Check sheet for the modelled part. Datum: model origin and axes. Units: mm. A direction names the side the tool comes from. Round coordinates to 2 decimals unless told otherwise and drop trailing zeros. Loops run counter-clockwise (first coordinate to the right, second up) from the corner with the lowest first, then second, coordinate; pieces in that order, holes last. Notation, with made-up numbers: (5, 47) - (31, 47) arc R26 ccw to (31, 64) - close; hole circle Ø4 at (85, 28.5). An arc over 180 degrees is marked (long way). Put each result on its own line as item: value.
```python
from build123d import *

# Parameters (mm, degrees)
SKETCH043_R     = 19
PAD026_DEPTH    = 3
PAD027_DEPTH    = 18.5
SKETCH045_W     = 5.4
SKETCH045_H     = 2
PAD028_DEPTH    = 1
SKETCH046_W     = 5.4
SKETCH046_H     = 2
PAD029_DEPTH    = 1
SKETCH047_W     = 5.4
SKETCH047_H     = 2
PAD030_DEPTH    = 1
SKETCH048_W     = 5.4
SKETCH048_H     = 2
PAD031_DEPTH    = 1
POCKET017_DEPTH = 5
CHAMFER_SIZE    = 1
CHAMFER001_SIZE = 1
CHAMFER002_SIZE = 1
CHAMFER003_SIZE = 1


with BuildPart() as part:
    # Sketch043 (on Face61 of Binder008) → Pad026 (new body)
    with BuildSketch(Plane.XY.offset(16.2)):
        with Locations((-83.63961, 83.63961)):
            Circle(SKETCH043_R)
    extrude(amount=PAD026_DEPTH)

    # Sketch044 (on Face2 of Pad026) → Pad027 (join)
    with BuildSketch(Plane(origin=(0, 0, 16.2), x_dir=(1, 0, 0), z_dir=(0, 0, -1))):
        Polygon((-92.9027091403, -78.1948880917), (-91.2056528655, -79.8919443665), (-87.3872762471, -76.0735677481), (-89.0843325219, -74.3765114732), align=None)
        Polygon((-79.8919443665, -76.0735677481), (-76.0735677481, -79.8919443665), (-74.3764965771, -78.1949029878), (-78.1948880917, -74.3765114732), align=None)
        Polygon((-92.9027199513, -89.0843217109), (-91.2056528655, -87.3872762471), (-87.3872762471, -91.2056528655), (-89.0843325219, -92.9027091403), align=None)
        Polygon((-79.8919443665, -91.2056528655), (-76.0735677481, -87.3872762471), (-74.3765262449, -89.0843472936), (-78.1948880917, -92.9027091403), align=None)
    extrude(amount=PAD027_DEPTH)

    # Sketch045 (on Face6 of Pad027) → Pad028 (join)
    with BuildSketch(Plane(origin=(-5.6568542495, -5.6568542495, 0), x_dir=(-0.7071067812, 0.7071067812, 0), z_dir=(0.7071067812, 0.7071067812, 0))):
        with Locations((118.2842712475, -1.3)):
            Rectangle(SKETCH045_W, SKETCH045_H)
    extrude(amount=PAD028_DEPTH)

    # Sketch046 (on Face11 of Pad028) → Pad029 (join)
    with BuildSketch(Plane(origin=(-89.2964645563, 89.2964645563, 0), x_dir=(0.7071067812, 0.7071067812, 0), z_dir=(0.7071067812, -0.7071067812, 0))):
        with Locations((0, -1.3)):
            Rectangle(SKETCH046_W, SKETCH046_H)
    extrude(amount=PAD029_DEPTH)

    # Sketch047 (on Face11 of Pad029) → Pad030 (join)
    with BuildSketch(Plane(origin=(-77.9827560573, 77.9827560573, 0), x_dir=(-0.7071067812, -0.7071067812, 0), z_dir=(-0.7071067812, 0.7071067812, 0))):
        with Locations((0, -1.3)):
            Rectangle(SKETCH047_W, SKETCH047_H)
    extrude(amount=PAD030_DEPTH)

    # Sketch048 (on Face15 of Pad030) → Pad031 (join)
    with BuildSketch(Plane(origin=(5.6568542495, 5.6568542495, 0), x_dir=(0.7071067812, -0.7071067812, 0), z_dir=(-0.7071067812, -0.7071067812, 0))):
        with Locations((-118.2842712475, -1.3)):
            Rectangle(SKETCH048_W, SKETCH048_H)
    extrude(amount=PAD031_DEPTH)

    # Sketch049 (on Face3 of Pad031) → Pocket017 (cut)
    with BuildSketch(Plane.XY.offset(19.2)):
        Polygon((-86.0396103068, 96.0396103068), (-81.2396103068, 96.0396103068), (-81.2396103068, 86.0396103068), (-71.2396103068, 86.0396103068), (-71.2396103068, 81.2396103068), (-81.2396103068, 81.2396103068), (-81.2396103068, 71.2396103068), (-86.0396103068, 71.2396103068), (-86.0396103068, 81.2396103068), (-96.0396103068, 81.2396103068), (-96.0396103068, 86.0396103068), (-86.0396103068, 86.0396103068), align=None)
    extrude(amount=-POCKET017_DEPTH, mode=Mode.SUBTRACT)

    # Chamfer
    chamfer_edges = [part.edges().sort_by_distance(p)[0] for p in [
        (-88.589358, 88.589358, -2.3),
    ]]
    chamfer(chamfer_edges, length=CHAMFER_SIZE)

    # Chamfer001
    chamfer001_edges = [part.edges().sort_by_distance(p)[0] for p in [
        (-78.689863, 88.589358, -2.3),
    ]]
    chamfer(chamfer001_edges, length=CHAMFER001_SIZE)

    # Chamfer002
    chamfer002_edges = [part.edges().sort_by_distance(p)[0] for p in [
        (-88.589358, 78.689863, -2.3),
    ]]
    chamfer(chamfer002_edges, length=CHAMFER002_SIZE)

    # Chamfer003
    chamfer003_edges = [part.edges().sort_by_distance(p)[0] for p in [
        (-78.689863, 78.689863, -2.3),
    ]]
    chamfer(chamfer003_edges, length=CHAMFER003_SIZE)


solid = part.part
```
Item 1: Section check C-C on x = -84. Enter the section's corners in (y, z).
Filled sheet:
outline: (64.64, 16.2) - (71.24, 16.2) - (71.24, 19.2) - (64.64, 19.2) - close; (96.04, 16.2) - (102.64, 16.2) - (102.64, 19.2) - (96.04, 19.2) - close
Item 2: Thickness scan on line 1 (Y direction, x = -84, z = 17.5); line 2 (Z direction, x = -88.5, y = 69.5); line 3 (Y direction, x = -78.5, z = 5). Record the ranges inside material, lowest first. Write a range as from..to.
Filled sheet:
line 1: 64.64..71.24, 96.04..102.64
line 2: 16.2..19.2
line 3: 74.68..77.47, 89.81..92.6
Item 3: Go/stop test with flat-tipped pins: pin 1 (1.5 mm diameter, centred on x = -78.5, z = 18, fed in from +Y); pin 2 (3.5 mm diameter, centred on y = 82.5, z = 18, fed in from +X); pin 3 (1.5 mm diameter, centred on y = 90.5, z = 3, fed in from -X); pin 4 (0.9 mm diameter, centred on x = -84, z = 18, fed in from +Y). Record where each tip stops, or that it passes through.
Filled sheet:
pin 1: y = 102.13
pin 2: x = -64.64
pin 3: x = -92.24
pin 4: y = 102.64
Item 4: Section check A-A on z = 11.5. Enter the section's corners in (x, y), then the cut area to 3 significant figures.
Filled sheet:
outline: (-92.9, 78.19) - (-89.08, 74.38) - (-87.39, 76.07) - (-91.21, 79.89) - close; (-92.9, 89.08) - (-91.21, 87.39) - (-87.39, 91.21) - (-89.08, 92.9) - close; (-79.89, 76.07) - (-78.19, 74.38) - (-74.38, 78.19) - (-76.07, 79.89) - close; (-79.89, 91.21) - (-76.07, 87.39) - (-74.38, 89.08) - (-78.19, 92.9) - close
area: 51.8 mm²
Item 5: Section check B-B on y = 90. Enter the section's corners in (x, z).
Filled sheet:
outline: (-101.54, 16.2) - (-91.99, 16.2) - (-91.99, -2.3) - (-88.59, -2.3) - (-87.18, -1.3) - (-87.18, -0.3) - (-88.59, -0.3) - (-88.59, 16.2) - (-86.04, 16.2) - (-86.04, 19.2) - (-101.54, 19.2) - close; (-81.24, 16.2) - (-78.69, 16.2) - (-78.69, -0.3) - (-80.1, -0.3) - (-80.1, -1.3) - (-78.69, -2.3) - (-75.29, -2.3) - (-75.29, 16.2) - (-65.74, 16.2) - (-65.74, 19.2) - (-81.24, 19.2) - close
Item 6: Section check D-D on y = 79. Enter the section's corners in (x, z), then the cut area to 3 significant figures.
Filled sheet:
outline: (-102.06, 16.2) - (-92.1, 16.2) - (-92.1, -2.3) - (-90.31, -2.3) - (-88.9, -1.3) - (-88.9, -0.3) - (-90.31, -0.3) - (-90.31, 16.2) - (-86.04, 16.2) - (-86.04, 19.2) - (-102.06, 19.2) - close; (-81.24, 16.2) - (-76.97, 16.2) - (-76.97, -0.3) - (-78.38, -0.3) - (-78.38, -1.3) - (-76.97, -2.3) - (-75.18, -2.3) - (-75.18, 16.2) - (-65.21, 16.2) - (-65.21, 19.2) - (-81.24, 19.2) - close
area: 166 mm²
Item 7: Tool access check on faces 4 (the flat face through (-91, 81.24, 18)), 5 (the flat face through (-76.26, 76.31, 7.08)), 6 (the flat face through (-89, 89, -0.3)). Record the directions out of +Z, -Z, +X, -X, +Y, -Y that give a thin tool (end or side, any length) a straight path to the whole face; none if there is none.
Filled sheet:
face 4: +Z, -Z
face 5: -Z, +X, -Y
face 6: none
Item 8: Release check for a two-part mould opening along Z. For faces 1 (the flat face through (-88.96, 88.91, -1.79)), 2 (the flat face through (-78.3, 78.4, -0.3)), 3 (the flat face through (-88.6, 78.7, -0.8)) record: +Z half, -Z half, draft (parallel to the pull), parting line (faces both ways), or undercut.
Filled sheet:
face 1: -Z half
face 2: undercut
face 3: draft
